from build123d import *

# Parameters (mm, degrees)
SKETCH_1_R              = 1.6
EXTRUDE_16_DEPTH        = 2
SKETCH_2_R              = 1.6
CUT_EXTRUDE_M3_DEPTH    = 2
CUT_EXTRUDE_537_DEPTH   = 2
SKETCH_4_R              = 1.65
F_8XM3_DEPTH            = 2
CUT_EXTRUDE_62X70_DEPTH = 2


with BuildPart() as part:
    # 草图1 → 正八边形下板_外围16孔_无支脚孔 (new body)
    with BuildSketch(Plane.XY):
        Polygon((90, 37.279220614), (37.279220614, 90), (-37.279220614, 90), (-90, 37.279220614), (-90, -37.279220614), (-37.279220614, -90), (37.279220614, -90), (90, -37.279220614), align=None)
        with Locations((83, 0)):
            Circle(SKETCH_1_R, mode=Mode.SUBTRACT)
        with Locations((76.682001198, 31.762724886)):
            Circle(SKETCH_1_R, mode=Mode.SUBTRACT)
        with Locations((58.689862838, 58.689862838)):
            Circle(SKETCH_1_R, mode=Mode.SUBTRACT)
        with Locations((31.762724886, 76.682001198)):
            Circle(SKETCH_1_R, mode=Mode.SUBTRACT)
        with Locations((0, 83)):
            Circle(SKETCH_1_R, mode=Mode.SUBTRACT)
        with Locations((-31.762724886, 76.682001198)):
            Circle(SKETCH_1_R, mode=Mode.SUBTRACT)
        with Locations((-58.689862838, 58.689862838)):
            Circle(SKETCH_1_R, mode=Mode.SUBTRACT)
        with Locations((-76.682001198, 31.762724886)):
            Circle(SKETCH_1_R, mode=Mode.SUBTRACT)
        with Locations((-83, 0)):
            Circle(SKETCH_1_R, mode=Mode.SUBTRACT)
        with Locations((-76.682001198, -31.762724886)):
            Circle(SKETCH_1_R, mode=Mode.SUBTRACT)
        with Locations((-58.689862838, -58.689862838)):
            Circle(SKETCH_1_R, mode=Mode.SUBTRACT)
        with Locations((-31.762724886, -76.682001198)):
            Circle(SKETCH_1_R, mode=Mode.SUBTRACT)
        with Locations((0, -83)):
            Circle(SKETCH_1_R, mode=Mode.SUBTRACT)
        with Locations((31.762724886, -76.682001198)):
            Circle(SKETCH_1_R, mode=Mode.SUBTRACT)
        with Locations((58.689862838, -58.689862838)):
            Circle(SKETCH_1_R, mode=Mode.SUBTRACT)
        with Locations((76.682001198, -31.762724886)):
            Circle(SKETCH_1_R, mode=Mode.SUBTRACT)
        with Locations((-35, -35)):
            Circle(SKETCH_1_R, mode=Mode.SUBTRACT)
        with Locations((-35, 35)):
            Circle(SKETCH_1_R, mode=Mode.SUBTRACT)
        with Locations((35, -35)):
            Circle(SKETCH_1_R, mode=Mode.SUBTRACT)
        with Locations((35, 35)):
            Circle(SKETCH_1_R, mode=Mode.SUBTRACT)
        with Locations((-24, -82.5)):
            Circle(SKETCH_1_R, mode=Mode.SUBTRACT)
        with Locations((-24, 82.5)):
            Circle(SKETCH_1_R, mode=Mode.SUBTRACT)
        with Locations((24, -82.5)):
            Circle(SKETCH_1_R, mode=Mode.SUBTRACT)
        with Locations((24, 82.5)):
            Circle(SKETCH_1_R, mode=Mode.SUBTRACT)
    extrude(amount=EXTRUDE_16_DEPTH)

    # 草图2 → 左右摄像头铰链M3孔 (cut)
    with BuildSketch(Plane.XY):
        with Locations((-80, -22)):
            Circle(SKETCH_2_R)
        with Locations((-80, 22)):
            Circle(SKETCH_2_R)
        with Locations((80, -22)):
            Circle(SKETCH_2_R)
        with Locations((80, 22)):
            Circle(SKETCH_2_R)
    extrude(amount=CUT_EXTRUDE_M3_DEPTH, mode=Mode.SUBTRACT)

    # 草图3 → Cut-Extrude 537 (cut)
    with BuildSketch(Plane.XY):
        Polygon((24, 9.941125497), (9.941125497, 24), (-9.941125497, 24), (-24, 9.941125497), (-24, -9.941125497), (-9.941125497, -24), (9.941125497, -24), (24, -9.941125497), align=None)
        Polygon((-18, 46), (18, 46), (22, 50), (22, 64), (18, 68), (-18, 68), (-22, 64), (-22, 50), align=None)
        Polygon((-46, -18), (-46, 18), (-50, 22), (-64, 22), (-68, 18), (-68, -18), (-64, -22), (-50, -22), align=None)
        Polygon((18, -46), (-18, -46), (-22, -50), (-22, -64), (-18, -68), (18, -68), (22, -64), (22, -50), align=None)
        Polygon((46, 18), (46, -18), (50, -22), (64, -22), (68, -18), (68, 18), (64, 22), (50, 22), align=None)
        Polygon((-42, -42), (-54, -42), (-42, -54), align=None)
        Polygon((-42, 42), (-54, 42), (-42, 54), align=None)
        Polygon((42, -42), (54, -42), (42, -54), align=None)
        Polygon((42, 42), (54, 42), (42, 54), align=None)
    extrude(amount=CUT_EXTRUDE_537_DEPTH, mode=Mode.SUBTRACT)

    # 草图4 → 四向侧支脚上角座8xM3 (cut)
    with BuildSketch(Plane.XY):
        with Locations((-28, -62)):
            Circle(SKETCH_4_R)
        with Locations((-62, -28)):
            Circle(SKETCH_4_R)
        with Locations((28, -62)):
            Circle(SKETCH_4_R)
        with Locations((-62, 28)):
            Circle(SKETCH_4_R)
        with Locations((-28, 62)):
            Circle(SKETCH_4_R)
        with Locations((62, -28)):
            Circle(SKETCH_4_R)
        with Locations((28, 62)):
            Circle(SKETCH_4_R)
        with Locations((62, 28)):
            Circle(SKETCH_4_R)
    extrude(amount=F_8XM3_DEPTH, mode=Mode.SUBTRACT)

    # 草图6 → 飞控螺丝检修口_62x70 (cut)
    with BuildSketch(Plane.XY):
        Polygon((-29, -35), (29, -35), (31, -33), (31, 33), (29, 35), (-29, 35), (-31, 33), (-31, -33), align=None)
    extrude(amount=CUT_EXTRUDE_62X70_DEPTH, mode=Mode.SUBTRACT)


solid = part.part
Work out the finished part from the listing and answer in its coordinate system (mm). A direction names the side the tool comes from. Round coordinates to 2 decimals unless told otherwise and drop trailing zeros. Loops run counter-clockwise (first coordinate to the right, second up) from the corner with the lowest first, then second, coordinate; pieces in that order, holes last. Notation, with made-up numbers: (29, 20) - (52, 20) arc R33 ccw to (52, 57) - close; hole circle Ø1 at (31.5, 25). An arc over 180 degrees is marked (long way). Use one line per item in the form item = value. Start each with the question number.
(1) Flat-ended cylindrical pins translate along their axes: P1, Ø5, axis at x = -31.76, y = -76.68, coming from the +Z side; P2, Ø0.6, axis at y = -53.5, z = 1.5, coming from the +X side; P3, Ø1, axis at x = 56.5, z = 1, coming from the +Y side. Find the tip coordinate at first contact, or state that the pin passes through.
(2) Find section C-C on y = -73. Determine the outline of the cut face in (x, z), and give its area (3 significant figures).
(3) Which of the six approach directions +Z, -Z, +X, -X, +Y, -Y give full straight-line access (tool end or side, diameter ignored) to faces 4 (the face through (48, -48, 1)), 5 (the face through (63.27, -64.01, 0.99))?
(4) Determine the mould class of faces 1 (the face through (66, -20, 1)), 2 (the face through (-64.01, -63.27, 0.99)), 3 (the face through (64.01, 63.27, 0.99)) for opening direction X: +X half, -X half, draft (parallel to the pull), parting line (faces both ways), or undercut.
(5) Consider line 1 (Y direction, x = 14.5, z = 1.95); line 2 (X direction, y = -12, z = 1.1); line 3 (Y direction, x = -35, z = 0.65). Determine where each line is inside the solid, lowest interval first.
(6) Find section B-B on z = 0.9. Give the number of separate pieces and of enclosed holes in the cut face, and give its area (3 significant figures).
(7) Find section A-A on y = 5.5. Determine the outline of the cut face in (x, z), and give its area (3 significant figures).
Answer list:
q1.P1 = 2
q1.P2 = 74.08
q1.P3 = 71.28
q2.outline = (-54.28, 0) - (54.28, 0) - (54.28, 2) - (-54.28, 2) - close
q2.area = 217 mm^2
q3.face_4 = +Z, -Z
q3.face_5 = +Z, -Z, +X, -Y
q4.face_1 = undercut
q4.face_2 = -X half
q4.face_3 = +X half
q5.line_1 = -90 to -68, -46 to -35, 35 to 46, 68 to 90
q5.line_2 = -90 to -68, -46 to -31, 31 to 46, 68 to 90
q5.line_3 = -90 to -36.6, -33.4 to 33.4, 36.6 to 90
q6.separate_pieces = 1
q6.enclosed_holes = 45
q6.area = 18,200 mm^2
q7.outline = (-90, 0) - (-68, 0) - (-68, 2) - (-90, 2) - close; (-46, 0) - (-31, 0) - (-31, 2) - (-46, 2) - close; (31, 0) - (46, 0) - (46, 2) - (31, 2) - close; (68, 0) - (90, 0) - (90, 2) - (68, 2) - close
q7.area = 148 mm^2
